The model under review builds one solid part; all positions refer to its coordinate system, in mm. Face numbers are marked on the shaded views. A direction names the side the tool comes from. Round coordinates to 2 decimals unless told otherwise and drop trailing zeros. Loops run counter-clockwise (first coordinate to the right, second up) from the corner with the lowest first, then second, coordinate; pieces in that order, holes last. Notation, with made-up numbers: M 28.25,30 L 40.25,30 A32 ccw 40.25,56 Z; hole C 81.5,17 d2. An arc over 180 degrees is marked long. Answer as a JSON object with one key per item and string values. Group by question number.
Item 1: Consider section A-A (y = 24.5). Give the boundary of the cut face in (x, z).
Item 2: The part is to be moulded in two halves that separate along X. For the marked faces 3, 4 and 5, say which applies: +X half, -X half, draft (parallel to the pull), parting line (faces both ways), or undercut.
Item 3: Insertion check: P1, Ø0.8, axis at y = -4.5, z = -0.5, coming from the +X side (3 decimals); P2, Ø0.7, axis at y = 26, z = -13.5, coming from the +X side; P3, Ø1.5, axis at y = 19.5, z = 3.5, coming from the +X side. Each pin has a flat end and moves straight along its axis. Give the tip position at first contact, or say it passes through.
Item 4: To check wall thickness, follow line 1 (X direction, y = 0.2, z = 0); line 2 (X direction, y = 39.7, z = 0); line 3 (Y direction, x = 11.3, z = 0). State the ranges of each line that lie inside material, in increasing order.
Item 5: Tool access review of the marked faces 1 and 2: name each direction out of +Z, -Z, +X, -X, +Y, -Y from which nothing blocks a thin tool from reaching the whole face with its end or side.
Item 6: Consider section B-B (y = 3.5). Give the boundary of the cut face in (x, z), and give its area (3 significant figures).
```python
from build123d import *

# Parameters (mm, degrees)
ESBO_O1_R                = 13.6
RESSALTO_EXTRUS_O1_DEPTH = 37.2
ESBO_O2_R                = 4.8
RESSALTO_EXTRUS_O2_DEPTH = 2.6
ESBO_O3_R                = 4.55
CORTE_EXTRUS_O1_DEPTH    = 0.25
ESBO_O4_R                = 1
RESSALTO_EXTRUS_O3_DEPTH = 11.5
FILETE1_R                = 0.5
ESBO_O5_R                = 1.25
CORTE_EXTRUS_O2_DEPTH    = 2
ESBO_O6_R                = 1.25
CORTE_EXTRUS_O3_DEPTH    = 2
ESBO_O7_R                = 13.35
ESBO_O7_R_2              = 9.5
CORTE_EXTRUS_O4_DEPTH    = 0.25
FILETE2_R                = 0.2
RESSALTO_EXTRUS_O4_START = 2.2
ESBO_O8_R                = 4.8
RESSALTO_EXTRUS_O4_DEPTH = 2.2
CORTE_EXTRUS_O5_START    = -0.25
ESBO_O9_R                = 4.55
CORTE_EXTRUS_O5_DEPTH    = 0.25
RESSALTO_EXTRUS_O5_START = 2.3
ESBO_O10_R               = 1
RESSALTO_EXTRUS_O5_DEPTH = 2.3
FILETE3_R                = 0.5
FILETE4_R                = 1
ESBO_O11_W               = 1.5
ESBO_O11_H               = 4.5
RESSALTO_EXTRUS_O6_DEPTH = 1.5
ESBO_O12_W               = 0.25
ESBO_O12_H               = 2.8
RESSALTO_EXTRUS_O7_DEPTH = 6
ESBO_O13_R               = 0.75
CORTE_EXTRUS_O6_DEPTH    = 59.436402419
FILETE5_R                = 1
ESBO_O14_R               = 1
CORTE_EXTRUS_O7_DEPTH    = 2
CORTE_EXTRUS_O8_DEPTH    = 2
RESSALTO_EXTRUS_O8_START = -13
RESSALTO_EXTRUS_O8_DEPTH = 20


with BuildPart() as part:
    # Esboço1 → Ressalto-extrusão1 (new body)
    with BuildSketch(Plane(origin=(0, 0, 0), x_dir=(1, 0, 0), z_dir=(0, 1, 0))):
        with Locations(Location((0, 0, 0), (0, 0, 270))):
            Circle(ESBO_O1_R)
    extrude(amount=RESSALTO_EXTRUS_O1_DEPTH)

    # Esboço2 → Ressalto-extrusão2 (add)
    with BuildSketch(Plane(origin=(0, 37.2, 0), x_dir=(1, 0, 0), z_dir=(0, 1, 0))):
        with Locations(Location((0, 0, 0), (0, 0, 270))):
            Circle(ESBO_O2_R)
    extrude(amount=RESSALTO_EXTRUS_O2_DEPTH)

    # Esboço3 → Corte-extrusão1 (cut)
    with BuildSketch(Plane(origin=(0, 39.8, 0), x_dir=(1, 0, 0), z_dir=(0, 1, 0))):
        with Locations(Location((0, 0, 0), (0, 0, 270))):
            Circle(ESBO_O3_R)
    extrude(amount=-CORTE_EXTRUS_O1_DEPTH, mode=Mode.SUBTRACT)

    # Esboço4 → Ressalto-extrusão3 (add)
    with BuildSketch(Plane(origin=(0, 39.55, 0), x_dir=(1, 0, 0), z_dir=(0, 1, 0))):
        with Locations(Location((0, 0, 0), (0, 0, 270))):
            Circle(ESBO_O4_R)
    extrude(amount=RESSALTO_EXTRUS_O3_DEPTH)

    # Filete1
    filete1_edges = [part.edges().sort_by_distance(p)[0] for p in [
        (0, 51.05, -1),
    ]]
    fillet(filete1_edges, radius=FILETE1_R)

    # Esboço5 → Corte-extrusão2 (cut)
    with BuildSketch(Plane(origin=(0, 37.2, 0), x_dir=(1, 0, 0), z_dir=(0, 1, 0))):
        with Locations(Location((-8, 0, 0), (0, 0, 270))):
            Circle(ESBO_O5_R)
        with Locations(Location((8, 0, 0), (0, 0, 90))):
            Circle(ESBO_O5_R)
    extrude(amount=-CORTE_EXTRUS_O2_DEPTH, mode=Mode.SUBTRACT)

    # Esboço6 → Corte-extrusão3 (cut)
    with BuildSketch(Plane(origin=(0, 37.2, 0), x_dir=(1, 0, 0), z_dir=(0, 1, 0))):
        with Locations(Location((0, 10.5, 0), (0, 0, 270))):
            Circle(ESBO_O6_R)
    extrude(amount=-CORTE_EXTRUS_O3_DEPTH, mode=Mode.SUBTRACT)

    # Esboço7 → Corte-extrusão4 (cut)
    with BuildSketch(Plane.XZ):
        with Locations(Location((0, 0, 0), (0, 0, 270))):
            Circle(ESBO_O7_R)
        with Locations(Location((0, 0, 0), (0, 0, 270))):
            Circle(ESBO_O7_R_2, mode=Mode.SUBTRACT)
    extrude(amount=-CORTE_EXTRUS_O4_DEPTH, mode=Mode.SUBTRACT)

    # Filete2
    filete2_edges = [part.edges().sort_by_distance(p)[0] for p in [
        (0, 0, 9.5),
    ]]
    fillet(filete2_edges, radius=FILETE2_R)

    # Esboço8 → Ressalto-extrusão4 (add)
    with BuildSketch(Plane.XZ.offset(RESSALTO_EXTRUS_O4_START)):
        with Locations(Location((0, 0, 0), (0, 0, 90))):
            Circle(ESBO_O8_R)
    extrude(amount=-RESSALTO_EXTRUS_O4_DEPTH)

    # Esboço9 → Corte-extrusão5 (cut)
    with BuildSketch(Plane.XZ.offset(2.2).offset(CORTE_EXTRUS_O5_START)):
        with Locations(Location((0, 0, 0), (0, 0, 90))):
            Circle(ESBO_O9_R)
    extrude(amount=CORTE_EXTRUS_O5_DEPTH, mode=Mode.SUBTRACT)

    # Esboço10 → Ressalto-extrusão5 (add)
    with BuildSketch(Plane.XZ.offset(1.95).offset(RESSALTO_EXTRUS_O5_START)):
        with Locations(Location((0, 0, 0), (0, 0, 90))):
            Circle(ESBO_O10_R)
    extrude(amount=-RESSALTO_EXTRUS_O5_DEPTH)

    # Filete3
    filete3_edges = [part.edges().sort_by_distance(p)[0] for p in [
        (0, -4.25, -1),
    ]]
    fillet(filete3_edges, radius=FILETE3_R)

    # Filete4
    filete4_edges = [part.edges().sort_by_distance(p)[0] for p in [
        (0, 37.2, -13.6),
    ]]
    fillet(filete4_edges, radius=FILETE4_R)

    # Esboço11 → Ressalto-extrusão6 (add)
    with BuildSketch(Plane.XZ.offset(-0.25)):
        with Locations((-11.25, 0)):
            Rectangle(ESBO_O11_W, ESBO_O11_H)
        with Locations((11.25, 0)):
            Rectangle(ESBO_O11_W, ESBO_O11_H)
    extrude(amount=RESSALTO_EXTRUS_O6_DEPTH)

    # Esboço12 → Ressalto-extrusão7 (add)
    with BuildSketch(Plane.XZ.offset(1.25)):
        with Locations((-11.25, 0)):
            Rectangle(ESBO_O12_W, ESBO_O12_H)
        with Locations((11.25, 0)):
            Rectangle(ESBO_O12_W, ESBO_O12_H)
    extrude(amount=RESSALTO_EXTRUS_O7_DEPTH)

    # Esboço13 → Corte-extrusão6 (cut, through all)
    with BuildSketch(Plane.ZY.offset(11.375)):
        with Locations((0, -5.85)):
            Circle(ESBO_O13_R)
    extrude(amount=-CORTE_EXTRUS_O6_DEPTH, mode=Mode.SUBTRACT)

    # Filete5
    filete5_edges = [part.edges().sort_by_distance(p)[0] for p in [
        (-11.25, -7.25, 1.4),
        (-11.25, -7.25, -1.4),
        (11.25, -7.25, 1.4),
        (11.25, -7.25, -1.4),
    ]]
    fillet(filete5_edges, radius=FILETE5_R)

    # Esboço14 → Corte-extrusão7 (cut)
    with BuildSketch(Plane.XZ):
        with Locations(Location((1.302361333, 7.386058148, 0), (0, 0, 270))):
            Circle(ESBO_O14_R)
        with Locations(Location((-1.302361333, -7.386058148, 0), (0, 0, 270))):
            Circle(ESBO_O14_R)
    extrude(amount=-CORTE_EXTRUS_O7_DEPTH, mode=Mode.SUBTRACT)

    # Esboço15 → Corte-extrusão8 (cut)
    with BuildSketch(Plane.XZ):
        with BuildLine():
            ThreePointArc((-5.463694682, 6.511377767), (-6.962792376, 4.875399709), (-7.987387277, 2.907171218))
            ThreePointArc((-7.987387277, 2.907171218), (-7.688551038, 2.266314836), (-7.047694656, 2.565151075))
            ThreePointArc((-7.047694656, 2.565151075), (-6.143640332, 4.301823273), (-4.820907073, 5.745333323))
            ThreePointArc((-4.820907073, 5.745333323), (-4.759278656, 6.44974935), (-5.463694682, 6.511377767))
        make_face()
        with BuildLine():
            ThreePointArc((4.820907073, -5.745333323), (6.143640332, -4.301823273), (7.047694656, -2.565151075))
            ThreePointArc((7.047694656, -2.565151075), (7.688551038, -2.266314836), (7.987387277, -2.907171218))
            ThreePointArc((7.987387277, -2.907171218), (6.962792376, -4.875399709), (5.463694682, -6.511377767))
            ThreePointArc((5.463694682, -6.511377767), (4.759278656, -6.44974935), (4.820907073, -5.745333323))
        make_face()
    extrude(amount=-CORTE_EXTRUS_O8_DEPTH, mode=Mode.SUBTRACT)

    # Esboço17 → Ressalto-extrusão8 (add)
    with BuildSketch(Plane.XZ.offset(RESSALTO_EXTRUS_O8_START)):
        with BuildLine():
            Line((-1.4, -13.527749258), (-1.4, -14.130817386))
            ThreePointArc((-1.4, -14.130817386), (0, 14.2), (1.4, -14.130817386))
            Line((1.4, -14.130817386), (1.4, -13.527749258))
            ThreePointArc((1.4, -13.527749258), (0, 13.6), (-1.4, -13.527749258))
        make_face()
    extrude(amount=-RESSALTO_EXTRUS_O8_DEPTH)


solid = part.part
```
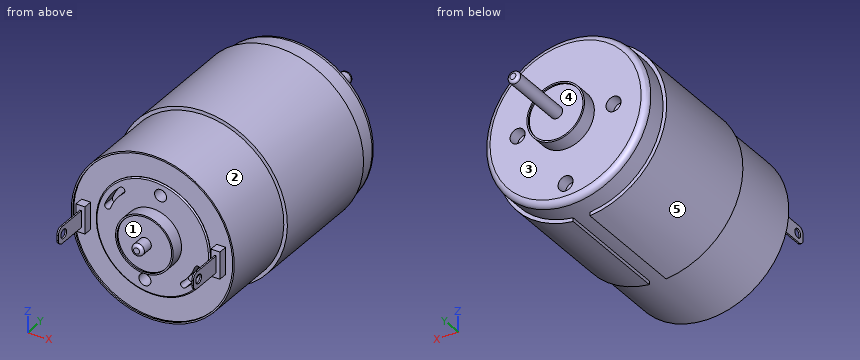
Geometry results:
{
 "1": {"outline": "M -1.4,-14.13 L -1.4,-13.53 A13.6 ccw 1.4,-13.53 L 1.4,-14.13 A14.2 ccw long Z"},
 "2": {"face 3": "draft", "face 4": "undercut", "face 5": "parting line"},
 "3": {"P1": "stops at x = 11.375", "P2": "stops at x = 5.36", "P3": "stops at x = 13.93"},
 "4": {"line 1": "x = -13.6 to -13.35, -12 to -10.5, -9.5 to 9.5, 10.5 to 12, 13.35 to 13.6", "line 2": "x = -4.8 to -4.55, -1 to 1, 4.55 to 4.8", "line 3": "y = -7.25 to -6.6, -5.1 to 37.2"},
 "5": {"face 1": "-Y", "face 2": "none"},
 "6": {"outline": "C 0,0 d27.2", "area": "581 mm^2"}
}
